```python
from build123d import *

# Parameters (mm, degrees)
F1_DEPTH = 12.7
F3_DEPTH = 2.54
F4_R     = 2.54


with BuildPart() as f1:
    # F0 (on Top) → F1 (new body)
    with BuildSketch(Plane.XY):
        with BuildLine():
            Line((-215.9, -101.6), (215.9, -101.6))
            ThreePointArc((215.9, -101.6), (227.059232, -74.659232), (254, -63.5))
            Line((254, -63.5), (254, 63.5))
            ThreePointArc((254, 63.5), (227.059232, 74.659232), (215.9, 101.6))
            Line((215.9, 101.6), (-215.9, 101.6))
            ThreePointArc((-215.9, 101.6), (-227.059232, 74.659232), (-254, 63.5))
            Line((-254, 63.5), (-254, -63.5))
            ThreePointArc((-254, -63.5), (-227.059232, -74.659232), (-215.9, -101.6))
        make_face()
    extrude(amount=-F1_DEPTH)

    # F2 (on face) → F3 (cut)
    with BuildSketch(Plane.XY):
        with BuildLine():
            ThreePointArc((241.3, 52.413112), (218.078976, 65.678976), (204.813112, 88.9))
            Line((204.813112, 88.9), (-204.813112, 88.9))
            ThreePointArc((-204.813112, 88.9), (-218.078976, 65.678976), (-241.3, 52.413112))
            Line((-241.3, 52.413112), (-241.3, -52.413112))
            ThreePointArc((-241.3, -52.413112), (-218.078976, -65.678976), (-204.813112, -88.9))
            Line((-204.813112, -88.9), (204.813112, -88.9))
            ThreePointArc((204.813112, -88.9), (218.078976, -65.678976), (241.3, -52.413112))
            Line((241.3, -52.413112), (241.3, 52.413112))
        make_face()
        with BuildLine():
            Line((-200.118461, 82.549997), (200.118461, 82.549997))
            ThreePointArc((200.118461, 82.549997), (213.588845, 61.188845), (234.949997, 47.718461))
            Line((234.949997, 47.718461), (234.949997, -47.718461))
            ThreePointArc((234.949997, -47.718461), (213.588845, -61.188845), (200.118461, -82.549997))
            Line((200.118461, -82.549997), (-200.118461, -82.549997))
            ThreePointArc((-200.118461, -82.549997), (-213.588845, -61.188845), (-234.949997, -47.718461))
            Line((-234.949997, -47.718461), (-234.949997, 47.718461))
            ThreePointArc((-234.949997, 47.718461), (-213.588845, 61.188845), (-200.118461, 82.549997))
        make_face(mode=Mode.SUBTRACT)
    extrude(amount=-F3_DEPTH, mode=Mode.SUBTRACT)

    # F4
    f4_edges = [f1.edges().sort_by_distance(p)[0] for p in [
        (-254, 63.5, -6.35),
        (-215.9, 101.6, -6.35),
        (254, 63.5, -6.35),
        (215.9, 101.6, -6.35),
        (254, -63.5, -6.35),
        (215.9, -101.6, -6.35),
        (-215.9, -101.6, -6.35),
        (-254, -63.5, -6.35),
    ]]
    fillet(f4_edges, radius=F4_R)


solid = f1.part
```
Check sheet for the modelled part. Datum: model origin and axes. Units: mm. A direction names the side the tool comes from. Round coordinates to 2 decimals unless told otherwise and drop trailing zeros. Order: outer loops, then holes, each group sorted by start corner. A loop starts at its lowest first (then second) coordinate and runs counter-clockwise, first axis right, second up. Notation, with made-up numbers: (83, 11.5) -> (131, 11.5) arc R31 cw to (131, 48.5) -> close; hole circle Ø6 at (-30, 12.5). An arc over 180 degrees is marked (long way). One line per item, written item: value. Start each with the question number.
Q1. Thickness scan on line 1 (Y direction, x = -34.5, z = -2.5); line 2 (X direction, y = -19, z = -2); line 3 (X direction, y = 77, z = -2.25). Record the ranges inside material, lowest first.
Q2. Set-up check for faces 1 (the face through (-3, -101.6, -6)), 2 (the face through (218.35, 65.41, -1.25)): record each of +Z, -Z, +X, -X, +Y, -Y from which the full face is reachable in a straight line by a thin tool's end or side.
Q3. Mould release check, pull along X, two halves, no side actions. Record for faces 3 (the face through (254, -1, -6)), 4 (the face through (-217.81, 65.95, -1.25)), 5 (the face through (-226.79, 74.93, -6.26)), 6 (the face through (3, 101.6, -6)): pulls with the +X half, pulls with the -X half, needs draft (parallel to the pull), parting line crosses it, or undercut.
Q4. Cross-section at A-A (z = -9.75). Record the boundary of the cut face in (x, y).
Q5. Gauge pin test, flat ends, axial feed: pin 1 Ø3 at (y, z) = (68, -8) entering from +X; pin 2 Ø6 at (y, z) = (73.5, -7.5) entering from -X; pin 3 Ø5 at (y, z) = (78.5, -6) entering from -X. Record the tip position at first contact, or that the pin passes through.
Completed:
1. line 1: y = -101.6 to -88.9, -82.55 to 82.55, 88.9 to 101.6
1. line 2: x = -254 to -241.3, -234.95 to 234.95, 241.3 to 254
1. line 3: x = -224.91 to -209.55, -202.42 to 202.42, 209.55 to 224.91
2. face 1: +Z, -Z, +X, -X, -Y
2. face 2: +Z
3. face 3: pulls with the +X half
3. face 4: undercut
3. face 5: pulls with the -X half
3. face 6: needs draft
4. outline: (-254, -61.04) arc R2.54 ccw to (-251.62, -63.57) arc R38.1 cw to (-215.97, -99.22) arc R2.54 ccw to (-213.44, -101.6) -> (213.44, -101.6) arc R2.54 ccw to (215.97, -99.22) arc R38.1 cw to (251.62, -63.57) arc R2.54 ccw to (254, -61.04) -> (254, 61.04) arc R2.54 ccw to (251.62, 63.57) arc R38.1 cw to (215.97, 99.22) arc R2.54 ccw to (213.44, 101.6) -> (-213.44, 101.6) arc R2.54 ccw to (-215.97, 99.22) arc R38.1 cw to (-251.62, 63.57) arc R2.54 ccw to (-254, 61.04) -> close
5. pin 1: stops at x = 239.18
5. pin 2: stops at x = -231.99
5. pin 3: stops at x = -225.78
